The listing builds one solid part. Answer for the finished solid, in the listing's coordinates (mm). Round coordinates to 2 decimals unless told otherwise and drop trailing zeros. Return JSON: item names as keys, results as strings. Group by question number.
(1) Find the intervals of material crossed by line 1 along Z through (x, y) = (-36, 303); line 2 along Z through (x, y) = (-19.05, 90); line 3 along Z through (x, y) = (-9, 239), in increasing order. Write a range as [from, to].
(2) Section A-A, the plane y = 385.5 is taken. Give the number of separate pieces and of enclosed holes in the cut face, then the cut area to 3 significant figures.
(3) Each of these flat-tipped pins is pushed along its axis until it touches: pin 1 (1 mm diameter, centred on x = -18.5, y = 338.5, fed in from -Z); pin 2 (4 mm diameter, centred on x = -7, z = -15.5, fed in from -Y). Where does it stop, or does it pass through?
(4) Determine the mould class of faces 1 (the flat face through (-4.267, 213, -65)), 2 (the flat face through (-33.833, 213, -12)), 3 (the flat face through (-11.989, 213, -57)), 4 (the flat face through (-7, 213, 0)) for opening direction X: +X half, -X half, draft (parallel to the pull), parting line (faces both ways), or undercut.
Autodesk Inventor part; units mm, degrees
ref_plane "YZ Plane" through (0, 0, 0) normal (1, 0, 0) x (0, 1, 0)
ref_plane "XZ Plane" through (0, 0, 0) normal (0, 1, 0) x (-1, 0, 0)
ref_plane "XY Plane" through (0, 0, 0) normal (0, 0, 1) x (1, 0, 0)
sketch "Sketch1" plane through (0, 0, 0) normal (0, 1, 0) x (-1, 0, 0)
  circle A0 centre (19.05, -19.05) radius 3.3274
  circle A1 centre (19.05, -57.15) radius 3.3274
  line L0 (0, 0) -> (15.0114, 0)
  line L1 (15.0114, 0) -> (15.0114, -4.2672)
  line L2 (15.0114, -4.2672) -> (8.001, -4.2672)
  line L3 (38.1, 0) -> (23.0886, 0)
  line L4 (23.0886, 0) -> (23.0886, -4.2672)
  line L5 (23.0886, -4.2672) -> (30.099, -4.2672)
  line L6 (23.0886, -11.0548) -> (15.0114, -11.0548)
  line L7 (30.099, -4.2672) -> (23.0886, -11.0548)
  line L8 (8.001, -4.2672) -> (15.0114, -11.0548)
  line L9 (38.1, 0) -> (38.1, -15.0114)
  line L10 (38.1, -15.0114) -> (33.8328, -15.0114)
  line L11 (33.8328, -15.0114) -> (33.8328, -8.001)
  line L12 (38.1, -76.2) -> (38.1, -61.1886)
  line L13 (38.1, -61.1886) -> (33.8328, -61.1886)
  line L14 (33.8328, -61.1886) -> (33.8328, -68.199)
  line L15 (38.1, -76.2) -> (23.0886, -76.2)
  line L16 (23.0886, -76.2) -> (23.0886, -71.9328)
  line L17 (23.0886, -71.9328) -> (30.099, -71.9328)
  line L18 (38.1, -23.0124) -> (38.1, -52.2224)
  line L19 (38.1, -23.0124) -> (33.8328, -23.0124)
  line L20 (33.8328, -23.0124) -> (33.8328, -30.0228)
  line L21 (38.1, -52.2224) -> (33.8328, -52.2224)
  line L22 (33.8328, -52.2224) -> (33.8328, -45.212)
  line L23 (26.1112, -15.0114) -> (26.1112, -23.0124)
  line L24 (26.1112, -52.2224) -> (26.1112, -61.1886)
  line L25 (33.8328, -8.001) -> (26.1112, -15.0114)
  line L26 (26.1112, -23.0124) -> (33.8328, -30.0228)
  line L27 (33.8328, -45.212) -> (26.1112, -52.2224)
  line L28 (26.1112, -61.1886) -> (33.8328, -68.199)
  line L29 (0, -76.2) -> (15.0114, -76.2)
  line L30 (15.0114, -76.2) -> (15.0114, -71.9328)
  line L31 (15.0114, -71.9328) -> (8.001, -71.9328)
  line L32 (23.0886, -64.2112) -> (15.0114, -64.2112)
  line L33 (15.0114, -64.2112) -> (8.001, -71.9328)
  line L34 (30.099, -71.9328) -> (23.0886, -64.2112)
  line L35 (0, 0) -> (0, -15.0114)
  line L36 (0, -15.0114) -> (4.2672, -15.0114)
  line L37 (4.2672, -15.0114) -> (4.2672, -8.001)
  line L38 (0, -76.2) -> (0, -61.1886)
  line L39 (0, -61.1886) -> (4.2672, -61.1886)
  line L40 (4.2672, -61.1886) -> (4.2672, -68.199)
  line L41 (11.9888, -15.0114) -> (11.9888, -23.0886)
  line L42 (11.9888, -15.0114) -> (4.2672, -8.001)
  line L43 (0, -22.3774) -> (0, -51.5874)
  line L44 (0, -51.5874) -> (4.2672, -51.5874)
  line L45 (4.2672, -51.5874) -> (4.2672, -44.577)
  line L46 (0, -22.3774) -> (4.2672, -22.3774)
  line L47 (4.2672, -22.3774) -> (4.2672, -29.3878)
  line L48 (4.2672, -29.3878) -> (11.9888, -23.0886)
  line L49 (11.9888, -61.1886) -> (11.9888, -53.1114)
  line L50 (4.2672, -68.199) -> (11.9888, -61.1886)
  line L51 (11.9888, -53.1114) -> (4.2672, -44.577)
  dimension "d0" = 38.1
  dimension "d1" = 76.2
  dimension "d2" = 6.6548
  dimension "d3" = 6.6548
  dimension "d8" = 15.0114
  dimension "d9" = 4.2672
  dimension "d10" = 7.0104
  dimension "d11" = 15.0114
  dimension "d12" = 4.2672
  dimension "d13" = 7.0104
  dimension "d14" = 15.0114
  dimension "d15" = 4.2672
  dimension "d16" = 7.0104
  dimension "d17" = 15.0114
  dimension "d18" = 4.2672
  dimension "d19" = 7.0104
  dimension "d20" = 15.0114
  dimension "d21" = 4.2672
  dimension "d22" = 7.0104
  dimension "d23" = 29.21
  dimension "d24" = 7.0104
  dimension "d25" = 4.2672
  dimension "d26" = 7.0104
  dimension "d27" = 8.001
  dimension "d28" = 11.9888
  dimension "d29" = 8.9662
  dimension "d32" = 11.9888
  dimension "d33" = 15.0114
  dimension "d34" = 4.2672
  dimension "d35" = 7.0104
  dimension "d36" = 11.9888
  dimension "d37" = 76.2
  dimension "d38" = 15.0114
  dimension "d39" = 4.2672
  dimension "d40" = 90
  dimension "d41" = 7.0104
  dimension "d42" = 15.0114
  dimension "d43" = 7.0104
  dimension "d44" = 8.0772
  dimension "d45" = 11.9888
  dimension "d46" = 29.21
  dimension "d47" = 7.0104
  dimension "d48" = 7.0104
  dimension "d49" = 8.0772
  dimension "d50" = 11.9888
extrude "Extrusion1" add sketch "Sketch1" along normal blind 431.8
properties part number "1530rail_17inch"
Working result:
{
 "1": {"line 1": "z = [-76.2, -61.19], [-52.22, -23.01], [-15.01, 0]", "line 2": "z = [-64.21, -60.48], [-53.82, -22.38], [-15.72, -11.05]", "line 3": "z = [-76.2, -71.93], [-70.83, -63.9], [-49.81, -25.53], [-12.3, -5.23], [-4.27, 0]"},
 "2": {"separate pieces": "1", "enclosed holes": "2", "area": "1,930 mm^2"},
 "3": {"pin 1": "stops at z = -64.21", "pin 2": "passes through"},
 "4": {"face 1": "undercut", "face 2": "undercut", "face 3": "+X half", "face 4": "draft"}
}
